Source: three-view drawing plus pictorial views. Frame: mm from the lowest corner of the part. A direction names the side the tool comes from. Give positions to 0.01 mm unless a question says otherwise; leave off trailing zeros. Loops run counter-clockwise (first coordinate to the right, second up) from the corner with the lowest first, then second, coordinate; pieces in that order, holes last. Notation, with made-up numbers: M -19.75,-14 L -8.75,-14 A21 cw -8.75,-2 Z; hole C -35,4 d11. An arc over 180 degrees is marked long. Answer as a JSON object with one key per item and string values. Group by question number.
1) Ray query, L1, parallel to X at y = 5.5, z = 1.8 (1 decimal); L2, parallel to Y at x = 9.5, z = 2.9; L3, parallel to X at y = 9.75, z = 3.05. Return the intervals inside material, ascending.
2) Section query A-A on y = 15. Return loops of the section in (x, z).
3) Section query D-D on z = 3.4. Return loops of the section in (x, y), plus the area to 3 significant figures.
4) Access query for the marked faces 1 and 2. Directions: +Z, -Z, +X, -X, +Y, -Y. A direction counts if a zero-diameter tool reaches every point of the face in a straight line with its end or side. Return the directions, or none.
5) Section query C-C on y = 6.5. Return loops of the section in (x, z), plus the area to 3 significant figures.
6) Section query B-B on x = 9.5. Return loops of the section in (y, z).
7) First-contact query: P1, Ø2, axis at y = 4, z = 3.5, coming from the +X side; P2, Ø3, axis at x = 3.5, z = 1.5, coming from the -Y side; P3, Ø1.3, axis at x = 4.3, y = 6.5, coming from the +Z side; P4, Ø1.5, axis at y = 3, z = 1, coming from the -X side. Flat tips, straight axial feed; report the tip coordinate or a pass-through.
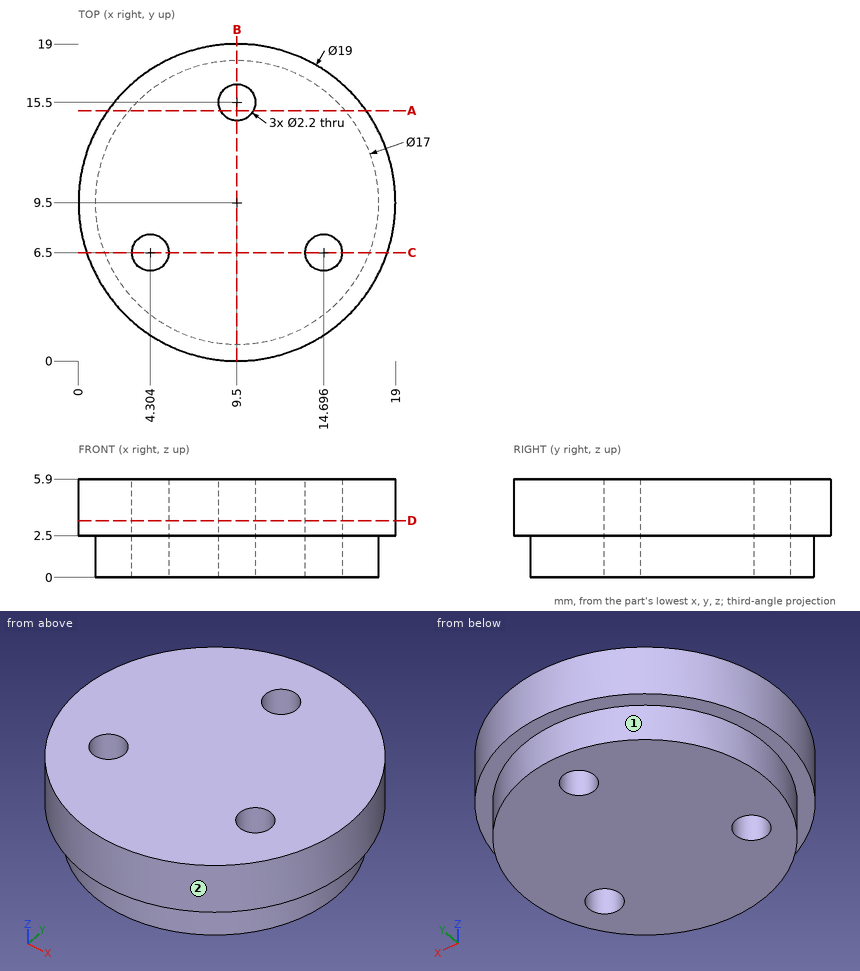
Output:
{
 "1": {"L1": "x = 2 to 3.8, 4.8 to 14.2, 15.2 to 17", "L2": "y = 0 to 14.4, 16.6 to 19", "L3": "x = 0 to 19"},
 "2": {"outline": "M 1.75,2.5 L 3.02,2.5 L 3.02,0 L 8.52,0 L 8.52,5.9 L 1.75,5.9 Z; M 10.48,0 L 15.98,0 L 15.98,2.5 L 17.25,2.5 L 17.25,5.9 L 10.48,5.9 Z"},
 "3": {"outline": "C 9.5,9.5 d19; hole C 4.3,6.5 d2.2; hole C 9.5,15.5 d2.2; hole C 14.7,6.5 d2.2", "area": "272 mm^2"},
 "4": {"face 1": "-Z", "face 2": "+Z, -Z"},
 "5": {"outline": "M 0.49,2.5 L 1.55,2.5 L 1.55,0 L 3.2,0 L 3.2,5.9 L 0.49,5.9 Z; M 5.4,0 L 13.6,0 L 13.6,5.9 L 5.4,5.9 Z; M 15.8,0 L 17.45,0 L 17.45,2.5 L 18.51,2.5 L 18.51,5.9 L 15.8,5.9 Z", "area": "75.1 mm^2"},
 "6": {"outline": "M 0,2.5 L 1,2.5 L 1,0 L 14.4,0 L 14.4,5.9 L 0,5.9 Z; M 16.6,0 L 18,0 L 18,2.5 L 19,2.5 L 19,5.9 L 16.6,5.9 Z"},
 "7": {"P1": "stops at x = 17.87", "P2": "stops at y = 1.35", "P3": "passes through", "P4": "stops at x = 3.24"}
}
